Build history of the part. All positions in model axes, mm. A direction names the side the tool comes from. Coordinates: 2 decimals unless noted, no trailing zeros. Order: outer loops, then holes, each group sorted by start corner. A loop starts at its lowest first (then second) coordinate and runs counter-clockwise, first axis right, second up. Notation, with made-up numbers: (49, 49) - (66, 49) arc R34 cw to (66, 84) - close; hole circle Ø6 at (16, 77.5). An arc over 180 degrees is marked (long way). Write each question's results on one line, items separated by ' | '. Start each with the question number.
from build123d import *

# Parameters (mm, degrees)
SKETCH_1_R           = 16
EXTRUDE_1_DEPTH      = 100
EXTRUDE_START        = -18
SKETCH_2_R           = 16
EXTRUDE_2_DEPTH      = 18
SKETCH_3_R           = 16
EXTRUDE_3_DEPTH      = 132
SKETCH_4_R           = 16
EXTRUDE_4_DEPTH      = 18
SKETCH_5_R           = 16
EXTRUDE_5_DEPTH      = 50
SKETCH_6_R           = 16
EXTRUDE_6_DEPTH      = 80
SKETCH_7_R           = 16
EXTRUDE_7_DEPTH      = 50
SKETCH_9_R           = 8
EXTRUDE_8_DEPTH      = 20
SKETCH_13_R          = 8
CUT_EXTRUDE_5_DEPTH  = 450
SKETCH_14_R          = 16
SKETCH_14_R_2        = 12.5
CUT_EXTRUDE_6_DEPTH  = 30
SKETCH_16_R          = 16
SKETCH_16_R_2        = 15
CUT_EXTRUDE_8_DEPTH  = 30
SKETCH_17_R          = 16
SKETCH_17_R_2        = 15
CUT_EXTRUDE_9_DEPTH  = 60
CUT_EXTRUDE_START    = -200
SKETCH_18_R          = 16
CUT_EXTRUDE_10_DEPTH = 200
CUT_EXTRUDE_START_2  = -20
SKETCH_19_R          = 16
SKETCH_19_R_2        = 8
CUT_EXTRUDE_11_DEPTH = 20
SKETCH_20_R          = 15
SKETCH_20_R_2        = 8
EXTRUDE_9_DEPTH      = 100
CUT_EXTRUDE_START_3  = -10
CUT_EXTRUDE_12_DEPTH = 10
CUT_EXTRUDE_START_4  = -12
SKETCH_22_R          = 15
SKETCH_22_R_2        = 11
CUT_EXTRUDE_13_DEPTH = 12


with BuildPart() as part:
    # 草图1 → 凸台-拉伸1 (new body)
    with BuildSketch(Plane(origin=(0, 0, 0), x_dir=(0, 0, -1), z_dir=(1, 0, 0))):
        Circle(SKETCH_1_R)
    extrude(amount=EXTRUDE_1_DEPTH)

    # 草图2 → 凸台-拉伸2 (add)
    with BuildSketch(Plane(origin=(100, 0, 0), x_dir=(0, 0, -1), z_dir=(1, 0, 0)).offset(EXTRUDE_START)):
        Circle(SKETCH_2_R)
    extrude(amount=EXTRUDE_2_DEPTH)

    # 草图3 → 凸台-拉伸3 (add)
    with BuildSketch(Plane(origin=(100, 0, 0), x_dir=(0, 0, -1), z_dir=(1, 0, 0))):
        Circle(SKETCH_3_R)
    extrude(amount=EXTRUDE_3_DEPTH)

    # 草图4 → 凸台-拉伸4 (add)
    with BuildSketch(Plane(origin=(232, 0, 0), x_dir=(0, 0, -1), z_dir=(1, 0, 0))):
        Circle(SKETCH_4_R)
    extrude(amount=EXTRUDE_4_DEPTH)

    # 草图5 → 凸台-拉伸5 (add)
    with BuildSketch(Plane(origin=(250, 0, 0), x_dir=(0, 0, -1), z_dir=(1, 0, 0))):
        Circle(SKETCH_5_R)
    extrude(amount=EXTRUDE_5_DEPTH)

    # 草图6 → 凸台-拉伸6 (add)
    with BuildSketch(Plane(origin=(300, 0, 0), x_dir=(0, 0, -1), z_dir=(1, 0, 0))):
        Circle(SKETCH_6_R)
    extrude(amount=EXTRUDE_6_DEPTH)

    # 草图7 → 凸台-拉伸7 (add)
    with BuildSketch(Plane(origin=(380, 0, 0), x_dir=(0, 0, -1), z_dir=(1, 0, 0))):
        Circle(SKETCH_7_R)
    extrude(amount=EXTRUDE_7_DEPTH)

    # 草图9 → 凸台-拉伸8 (add)
    with BuildSketch(Plane(origin=(430, 0, 0), x_dir=(0, 0, -1), z_dir=(1, 0, 0))):
        Circle(SKETCH_9_R)
    extrude(amount=EXTRUDE_8_DEPTH)

    # 草图13 → 切除-拉伸5 (cut)
    with BuildSketch(Plane.ZY):
        Circle(SKETCH_13_R)
    extrude(amount=-CUT_EXTRUDE_5_DEPTH, mode=Mode.SUBTRACT)

    # 草图14 → 切除-拉伸6 (cut)
    with BuildSketch(Plane.ZY):
        Circle(SKETCH_14_R)
        Circle(SKETCH_14_R_2, mode=Mode.SUBTRACT)
    extrude(amount=-CUT_EXTRUDE_6_DEPTH, mode=Mode.SUBTRACT)

    # 草图16 → 切除-拉伸8 (cut)
    with BuildSketch(Plane.ZY.offset(-30)):
        Circle(SKETCH_16_R)
        Circle(SKETCH_16_R_2, mode=Mode.SUBTRACT)
    extrude(amount=-CUT_EXTRUDE_8_DEPTH, mode=Mode.SUBTRACT)

    # 草图17 → 切除-拉伸9 (cut)
    with BuildSketch(Plane.ZY.offset(-160)):
        Circle(SKETCH_17_R)
        Circle(SKETCH_17_R_2, mode=Mode.SUBTRACT)
    extrude(amount=-CUT_EXTRUDE_9_DEPTH, mode=Mode.SUBTRACT)

    # 草图18 → 切除-拉伸10 (cut)
    with BuildSketch(Plane(origin=(430, 0, 0), x_dir=(0, 0, -1), z_dir=(1, 0, 0)).offset(CUT_EXTRUDE_START)):
        with Locations(Location((0, 0, 0), (0, 0, 180))):
            Circle(SKETCH_18_R)
    extrude(amount=CUT_EXTRUDE_10_DEPTH, mode=Mode.SUBTRACT)

    # 草图19 → 切除-拉伸11 (cut)
    with BuildSketch(Plane(origin=(230, 0, 0), x_dir=(0, 0, -1), z_dir=(1, 0, 0)).offset(CUT_EXTRUDE_START_2)):
        with Locations(Location((0, 0, 0), (0, 0, 180))):
            Circle(SKETCH_19_R)
        with Locations(Location((0, 0, 0), (0, 0, 180))):
            Circle(SKETCH_19_R_2, mode=Mode.SUBTRACT)
    extrude(amount=CUT_EXTRUDE_11_DEPTH, mode=Mode.SUBTRACT)

    # 草图20 → 凸台-拉伸9 (add)
    with BuildSketch(Plane(origin=(210, 0, 0), x_dir=(0, 0, -1), z_dir=(1, 0, 0))):
        with Locations(Location((0, 0, 0), (0, 0, 180))):
            Circle(SKETCH_20_R)
        with Locations(Location((0, 0, 0), (0, 0, 180))):
            Circle(SKETCH_20_R_2, mode=Mode.SUBTRACT)
    extrude(amount=EXTRUDE_9_DEPTH)

    # 草图21 → 切除-拉伸12 (cut)
    with BuildSketch(Plane(origin=(200, 0, 0), x_dir=(0, 0, -1), z_dir=(1, 0, 0)).offset(CUT_EXTRUDE_START_3)):
        with BuildLine():
            Line((-15, 0), (-8, 0))
            ThreePointArc((-8, 0), (-5.656854249, 5.656854249), (0, 8))
            Line((0, 8), (0, 15))
            ThreePointArc((0, 15), (-10.606601718, 10.606601718), (-15, 0))
        make_face()
        with BuildLine():
            Line((8, 0), (15, 0))
            ThreePointArc((15, 0), (10.606601718, -10.606601718), (0, -15))
            Line((0, -15), (0, -8))
            ThreePointArc((0, -8), (5.656854249, -5.656854249), (8, 0))
        make_face()
    extrude(amount=CUT_EXTRUDE_12_DEPTH, mode=Mode.SUBTRACT)

    # 草图22 → 切除-拉伸13 (cut)
    with BuildSketch(Plane(origin=(310, 0, 0), x_dir=(0, 0, -1), z_dir=(1, 0, 0)).offset(CUT_EXTRUDE_START_4)):
        with Locations(Location((0, 0, 0), (0, 0, 180))):
            Circle(SKETCH_22_R)
        Circle(SKETCH_22_R_2, mode=Mode.SUBTRACT)
    extrude(amount=CUT_EXTRUDE_13_DEPTH, mode=Mode.SUBTRACT)


solid = part.part
Item 1: Slice it at A-A (y = 4). Write the cut outline in (x, z), then the cut area to 3 significant figures.
Item 2: Probe probe 1 along X at (y, z) = (-7, -5.5); probe 2 along Y at (x, z) = (213, 1); probe 3 along Y at (x, z) = (126.5, 0). List the from-to ranges inside material, lowest first.
Item 3: Which spindle directions (+Z, -Z, +X, -X, +Y, -Y) get a long thin tool onto all of the face, cutting with end or side? Do faces 5 (the flat face through (200, 8, 8)), 6 (the flat face through (195, -12, 0)), 7 (the cylindrical face through (109.3, -15.62, 3.47)), 8 (the cylindrical face through (44.79, 0.66, -14.985)), 9 (the flat face through (0, -8.2, 0.2)). Say none if no direction does.
Item 4: Pull direction X, two halves, no side cores. Call faces 1 (the flat face through (298, -10, -5)), 2 (the flat face through (195, 0, 12)), 3 (the cylindrical face through (303.92, -10.74, 2.38)), 4 (the flat face through (30, 12.3, -3.4)): released by +X, released by -X, zero draft, split by the parting line, or undercut.
Item 5: Slice it at C-C (x = 143). Write the cut outline in (y, z), then the cut area to 3 significant figures.
Item 6: Flat gauge pins, fed straight in: P1, Ø5.5, axis at x = 194, y = -13, coming from the -Z side; P2, Ø2, axis at x = 194.5, y = 10.5, coming from the +Z side; P3, Ø7.5, axis at x = 196, z = -11, coming from the -Y side. Where does each tip first touch, or does it go through?
Item 7: Slice it at B-B (x = 256.5). Write the cut outline in (y, z), then the cut area to 3 significant figures.
Resolved:
1) outline: (0, -11.84) - (30, -11.84) - (30, -14.46) - (60, -14.46) - (60, -15.49) - (160, -15.49) - (160, -14.46) - (298, -14.46) - (298, -10.25) - (310, -10.25) - (310, -6.93) - (0, -6.93) - close; (0, 6.93) - (190, 6.93) - (190, 14.46) - (160, 14.46) - (160, 15.49) - (60, 15.49) - (60, 14.46) - (30, 14.46) - (30, 11.84) - (0, 11.84) - close; (200, 6.93) - (310, 6.93) - (310, 10.25) - (298, 10.25) - (298, 14.46) - (200, 14.46) - close | area: 4,540 mm^2
2) probe 1: 0 to 190, 200 to 310 | probe 2: -14.97 to -7.94, 7.94 to 14.97 | probe 3: -16 to -8, 8 to 16
3) face 5: +Z, +Y | face 6: -Z, -Y | face 7: +X, -X | face 8: -X | face 9: +Z, -Z, -X, +Y, -Y
4) face 1: released by +X | face 2: undercut | face 3: zero draft | face 4: released by -X
5) outline: circle Ø32 at (0, 0); hole circle Ø16 at (0, 0) | area: 603 mm^2
6) P1: z = 0 | P2: z = 0 | P3: y = 0
7) outline: circle Ø30 at (0, 0); hole circle Ø16 at (0, 0) | area: 506 mm^2
